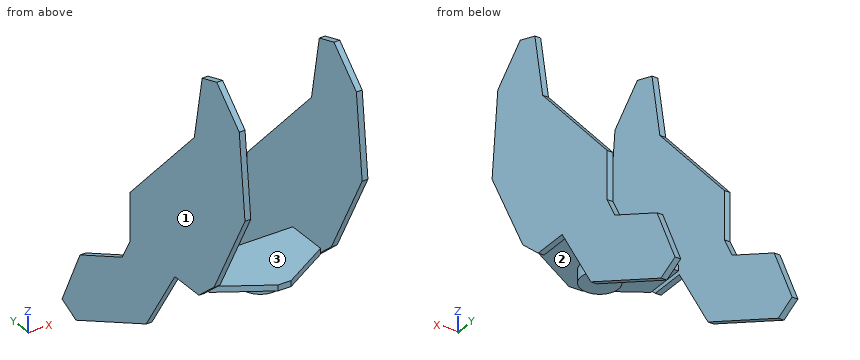
Autodesk Inventor part; units mm, degrees
ref_plane "Work Plane1" through (-24.1297, -20.1241, 6.985) normal (0, 0, -1) x (0, 1, 0)
ref_plane "Work Plane2" through (-24.1297, -20.1241, 10.16) normal (0, 0, 1) x (1, 0, 0)
ref_plane "Work Plane4" through (-33.6547, -38.1116, -58.8269) normal (-1, 0, 0) x (0, 0.0012, 1)
sketch "Sketch1" plane through (0, 0, 0) normal (0, 0, 1) x (1, 0, 0)
  circle A0 centre (0, 0) radius 10.16
  arc A1 (-9.6844, 3.0721) -> (-9.6844, -3.0721) centre (0, 0) ccw construction
ref_plane "Work Plane1" through (-24.1297, -20.1241, 6.985) normal (0, 0, -1) x (0, 1, 0)
extrude "Extrusion1" add sketch "Sketch1" along normal up to surface (6.985 mm away)
sketch "Sketch2" plane through (0, 0, 6.985) normal (0, 0, 1) x (1, 0, 0)
  line L0 (-24.1297, 19.05) -> (24.1297, 19.05) construction
  line L1 (-30.4797, 4.9571) -> (-30.4797, 51.5313) construction
  line L2 (30.4797, 51.5313) -> (30.4797, 4.9571) construction
  line L3 (-3.5464, -20.1241) -> (3.5464, -20.1241)
  line L4 (3.5464, -20.1241) -> (30.4797, -3.81)
  line L5 (-3.5464, -20.1241) -> (-30.4797, -3.81)
  line L6 (-30.4797, -3.81) -> (-30.4797, 19.05)
  line L7 (-30.4797, 19.05) -> (30.4797, 19.05)
  line L8 (30.4797, 19.05) -> (30.4797, -3.81)
  line L9 (0, 141.501) -> (0, -68.047)
  arc A0 (-6.5797, -18.2867) -> (6.5797, -18.2867) centre (0, -7.4241) ccw construction
  line L10 (-6.5797, -18.2867) -> (-24.1297, -7.6563) construction
  line L11 (24.1297, -7.6563) -> (6.5797, -18.2867) construction
  point P0 (0, 0)
  point P1 (0, -20.1241)
ref_plane "Work Plane2" through (-24.1297, -20.1241, 10.16) normal (0, 0, 1) x (1, 0, 0)
extrude "Extrusion2" add sketch "Sketch2" along normal up to surface (3.175 mm away)
ref_plane "Work Plane3" through (-30.4797, 28.613, 25.8435) normal (1, 0, 0) x (0, 1, -0.0012)
sketch "Sketch3" plane through (-30.4797, 28.613, 25.8435) normal (1, 0, 0) x (0, 1, -0.0012)
  line L0 (-60.3032, 83.7671) -> (-46.2664, 96.8991) construction
  line L1 (-40.061, 98.3138) -> (-35.1427, 96.7719) construction
  line L2 (-30.8232, 91.9054) -> (-25.3621, 62.7037) construction
  line L3 (-66.4956, 38.9741) -> (-62.271, 79.8043) construction
  line L4 (-41.8663, -9.4545) -> (-65.7822, 35.3495) construction
  line L5 (-23.7279, 59.5092) -> (22.9055, 10.5268) construction
  line L6 (28.1348, -2.5269) -> (28.1554, -19.5123) construction
  line L7 (-12.3805, -21.1807) -> (-26.3576, -21.2033) construction
  line L8 (-30.4769, -19.6947) -> (-40.5808, -11.1193) construction
  line L9 (13.7735, -56.6336) -> (-7.0203, -24.1102) construction
  line L10 (69.8762, -83.775) -> (16.4352, -58.9603) construction
  line L11 (28.9647, -22.6068) -> (33.5205, -30.7438) construction
  line L12 (36.3869, -33.401) -> (67.1857, -47.7021) construction
  line L13 (70.2201, -50.6979) -> (81.3231, -73.8278) construction
  line L14 (78.362, -82.2562) -> (75.2702, -83.7404) construction
  line L15 (-62.0279, 82.1535) -> (-43.5762, 99.4159)
  line L16 (-43.5762, 99.4159) -> (-31.521, 95.6364)
  line L17 (-31.521, 95.6364) -> (-25.0181, 60.8644)
  line L18 (-25.0181, 60.8644) -> (28.1257, 5.0437)
  line L19 (28.1257, 5.0437) -> (28.1574, -21.1648)
  line L20 (28.1574, -21.1648) -> (34.5239, -32.536)
  line L21 (34.5239, -32.536) -> (69.2399, -48.656)
  line L22 (69.2399, -48.656) -> (84.0568, -79.5226)
  line L23 (84.0568, -79.5226) -> (72.5814, -85.0311)
  line L24 (72.5814, -85.0311) -> (14.7653, -58.1848)
  line L25 (14.7653, -58.1848) -> (-8.8968, -21.1751)
  line L26 (-8.8968, -21.1751) -> (-28.6949, -21.2071)
  line L27 (-28.6949, -21.2071) -> (-41.3065, -10.5034)
  line L28 (-41.3065, -10.5034) -> (-66.6939, 37.0577)
  line L29 (-66.6939, 37.0577) -> (-62.0279, 82.1535)
  point P0 (-28.5817, -25.8781)
ref_plane "Work Plane4" through (-33.6547, -38.1116, -58.8269) normal (-1, 0, 0) x (0, 0.0012, 1)
extrude "Extrusion3" add sketch "Sketch3" against normal up to surface (3.175 mm away)
mirror "Mirror1" about plane through (0, 0, 0) normal (1, 0, 0) of "Extrusion3"
properties part number "ShoulderCollision"
Verification items for the finished model (mm, model axes). Face numbers are marked on the shaded views. A direction names the side the tool comes from. Round coordinates to 2 decimals unless told otherwise and drop trailing zeros. Order: outer loops, then holes, each group sorted by start corner. A loop starts at its lowest first (then second) coordinate and runs counter-clockwise, first axis right, second up.
1) Cross-section at D-D, the plane x = 15. Record the cut outline in (y, z) (3 decimals).
Geometry says:
outline: (-13.186, 6.985) - (19.05, 6.985) - (19.05, 10.16) - (-13.186, 10.16) - close
2) Tool access check on the marked faces 1, 2 and 3. Record the directions out of +Z, -Z, +X, -X, +Y, -Y that give a thin tool (end or side, any length) a straight path to the whole face; none if there is none.
Geometry says:
face 1: +Z, -Z, -X, +Y, -Y
face 2: -Z
face 3: +Z, +Y, -Y
3) Cross-section at C-C, the plane z = 102. Record the cut outline in (x, y).
Geometry says:
outline: (-33.65, -33.95) - (-30.48, -33.95) - (-30.48, 0.83) - (-33.65, 0.83) - close; (30.48, -33.95) - (33.65, -33.95) - (33.65, 0.83) - (30.48, 0.83) - close
4) Depth check by flat-ended pin: pin 1 (2.5 mm diameter, centred on x = -1.5, z = 8.5, fed in from -Y); pin 2 (5 mm diameter, centred on x = 19, y = -6.5, fed in from +Z); pin 3 (10 mm diameter, centred on x = -26.5, z = 68.5, fed in from -Y); pin 4 (0.7 mm diameter, centred on y = -3.5, z = 7.5, fed in from +X). Enter the tip coordinate at first touch or a pass-through.
Geometry says:
pin 1: stops at y = -20.12
pin 2: stops at z = 10.16
pin 3: stops at y = -37.78
pin 4: stops at x = 33.65
5) Cross-section at A-A, the plane y = 84.5. Record the cut outline in (x, z).
Geometry says:
outline: (-33.65, -51.55) - (-30.48, -51.55) - (-30.48, -16.7) - (-33.65, -16.7) - close; (30.48, -51.55) - (33.65, -51.55) - (33.65, -16.7) - (30.48, -16.7) - close
6) Material ranges on line 1 (X direction, y = 58.5, z = -33); line 2 (Z direction, x = -12, y = 4) (3 decimals); line 3 (Z direction, x = -31, y = -27), recorded low to high.
Geometry says:
line 1: x = -33.65 to -30.48, 30.48 to 33.65
line 2: z = 6.985 to 10.16
line 3: z = 42.25 to 113.97
7) Cross-section at B-B, the plane x = 0. Record the cut outline in (y, z) (3 decimals).
Geometry says:
outline: (-20.124, 6.985) - (-10.16, 6.985) - (-10.16, 0) - (10.16, 0) - (10.16, 6.985) - (19.05, 6.985) - (19.05, 10.16) - (-20.124, 10.16) - close
